Design review of the part built by this model. Coordinates are the model's own, in mm. Face numbers are marked on the shaded views. A direction names the side the tool comes from. Round coordinates to 2 decimals unless told otherwise and drop trailing zeros. Write each loop counter-clockwise with the first axis right and the second up, starting at its lowest first coordinate (ties: lowest second). Pieces come first, ordered by that corner, then holes. Notation, with made-up numbers: (-20.75, 44.5) -> (-15.75, 44.5) arc R28 ccw to (-15.75, 68.5) -> close; hole circle Ø4 at (-1, 55.25). An arc over 180 degrees is marked (long way). Write item = value, one per line. Start each with the question number.
Item 1: Add section A-A, the plane y = -7. State the section outline as (x, z) points.
Item 2: Machinability: for the marked faces 4, 5 and 6, which of the approach directions +Z, -Z, +X, -X, +Y, -Y give a long, thin tool a straight path to every point of the face, cutting with its end or side? Answer none if there is none.
Item 3: Add section C-C, the plane z = -124. State the section outline as (x, y) points, then the cut area to 3 significant figures.
Item 4: Add section B-B, the plane x = 213. State the section outline as (y, z) points.
Item 5: To check wall thickness, follow L1, parallel to Z at x = 251, y = 0; L2, parallel to Y at x = -15.5, z = -142.5; L3, parallel to Y at x = 222.5, z = -102. State the ranges of each line that lie inside material, in increasing order.
Item 6: Mouldability with a two-part tool opening along Z and no side actions: class the marked faces 1, 2 and 3 as released by +Z, released by -Z, zero draft, split by the parting line, or undercut.
Item 7: For pin 1 Ø1 at (y, z) = (-8.5, -175) entering from -X; pin 2 Ø3 at (x, y) = (177, 14.5) entering from +Z; pin 3 Ø3 at (y, z) = (3.5, -131.5) entering from -X, all flat-tipped, find the tip position at first contact; note any pin that passes through.
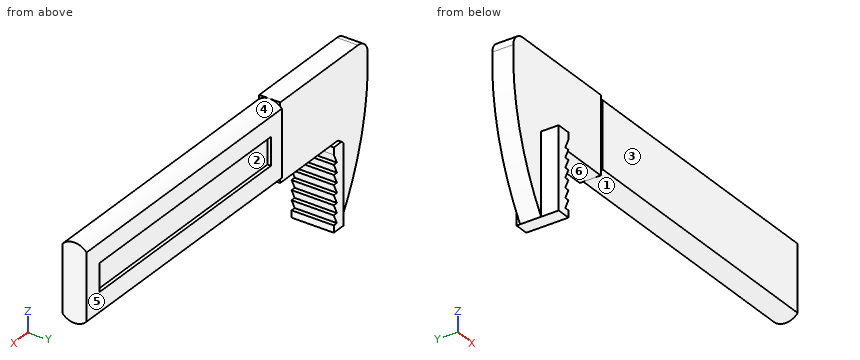
Autodesk Inventor part; units mm, degrees
ref_plane "YZ Plane" through (0, 0, 0) normal (1, 0, 0) x (0, 1, 0)
ref_plane "XZ Plane" through (0, 0, 0) normal (0, 1, 0) x (-1, 0, 0)
ref_plane "XY Plane" through (0, 0, 0) normal (0, 0, 1) x (1, 0, 0)
sketch "Sketch1" plane through (0, 0, 0) normal (0, 1, 0) x (-1, 0, 0)
  line L0 (0, -131.5012) -> (-0.0617, -190.607)
  line L1 (-41.7658, -131.5012) -> (53.7037, -131.5012) construction
  line L2 (28.2495, -75.6212) -> (-41.7658, -75.6212)
  arc A0 (-0.0617, -190.607) -> (28.2495, -75.6212) centre (-152.8189, -92.0177) ccw
  line L3 (28.2495, -75.6212) -> (-62.1692, -75.6212)
  line L4 (-62.1692, -75.6212) -> (-62.1692, -131.5012)
  line L5 (-62.1692, -131.5012) -> (0, -131.5012)
  point P0 (0, 0)
  point P1 (8.9112, -179.6369)
  point P2 (0, -75.6212)
  point P3 (-70.1734, -131.5012)
  dimension "d21" = 59.1058
  dimension "d37" = 70.0153
extrude "Extrusion1" add sketch "Sketch1" along normal blind 15.24
fillet "Fillet1" radius 10.16 1 edges at (-28.2495, 7.62, -75.6212)
sketch "Sketch4" plane through (0.0191, 12.7, -149.7788) normal (0.9999995, 0, 0.0010447) x (0.0010447, 0, -0.9999995)
  line L0 (0, -22.86) -> (0, 2.54)
  line L1 (15.9389, 2.54) -> (13.4561, 2.54) construction
  line L2 (13.4561, 2.54) -> (13.4561, 4.185) construction
  line L3 (13.6464, 2.54) -> (33.02, 2.54)
  line L4 (33.02, -22.86) -> (13.6464, -22.86)
  line L5 (-10.4713, -22.86) -> (-10.4713, 2.54) construction
  line L6 (-10.4713, -10.16) -> (33.02, -10.16) construction
  line L7 (-10.4713, -10.16) -> (11.2743, -10.16) construction
  line L8 (-18.2773, 5.1507) -> (40.826, 5.1507)
  line L9 (40.826, 5.1507) -> (40.826, -25.4707)
  line L10 (40.826, -25.4707) -> (-18.2773, -25.4707)
  line L11 (-18.2773, -25.4707) -> (-18.2773, 5.1507)
  line L12 (-18.2773, 5.1507) -> (40.826, -25.4707) construction
  line L13 (40.826, 5.1507) -> (-18.2773, -25.4707) construction
  point P0 (8.89, -10.16)
  dimension "d24" = 43.4913
  dimension "d23" = 21.7457
extrude "Extrusion4" add sketch "Sketch4" along normal blind 10.16
sketch "Sketch5" plane through (0, 17.8507, -131.5015) normal (0, 1, 0) x (0.9999995, 0, 0.0010447)
  line L0 (10.16, 0) -> (10.16, 59.1033)
  line L1 (10.16, 0) -> (10.16, 4.6168)
  line L2 (10.16, 0) -> (10.16, 6.604)
  line L3 (10.16, 59.1033) -> (10.16, 54.0318)
  line L4 (10.16, 54.0318) -> (6.8983, 54.0318)
  line L5 (6.8983, 54.0318) -> (10.16, 47.0371)
  line L6 (10.16, 3.5366) -> (10.16, 0)
  line L7 (10.16, 54.0318) -> (10.16, 59.1033)
  line L8 (10.16, 47.0371) -> (6.8983, 47.0371)
  line L9 (6.8983, 47.0371) -> (10.16, 40.0424)
  line L10 (10.16, 40.0424) -> (6.8983, 40.0424)
  line L11 (6.8983, 40.0424) -> (10.16, 33.0478)
  line L12 (10.16, 33.0478) -> (6.8983, 33.0478)
  line L13 (6.8983, 33.0478) -> (10.16, 26.0531)
  line L14 (10.16, 26.0531) -> (6.8983, 26.0531)
  line L15 (6.8983, 26.0531) -> (10.16, 19.0584)
  line L16 (10.16, 19.0584) -> (6.8983, 19.0584)
  line L17 (6.8983, 19.0584) -> (10.16, 12.0637)
  line L18 (10.16, 12.0637) -> (6.8983, 12.0637)
  line L19 (6.8983, 12.0637) -> (10.16, 5.0691)
  line L20 (10.16, 5.0691) -> (10.16, 54.0318)
  point P0 (-241.3, 27.1673)
  dimension "d30" = 5.0715
  dimension "d28" = 65
  dimension "d29" = 6.9947
extrude "Extrusion5" cut sketch "Sketch5" against normal through all
fillet "Fillet3" radius 3.175 1 edges at (0, 16.5453, -131.5015)
sketch "Sketch7" plane through (62.1692, 0, -75.6212) normal (1, 0, 0) x (0, 0, -1)
  line L0 (0, 15.24) -> (55.88, 15.24)
  line L1 (55.88, 0) -> (27.2823, 0)
  line L2 (27.94, 0) -> (41.91, 0) construction
  line L3 (55.88, 0) -> (55.88, 15.24)
  line L4 (55.88, 0) -> (27.94, 0)
  line L5 (9.7909, 0) -> (0, 0)
  line L6 (27.94, 0) -> (27.94, 15.24)
  line L7 (27.94, 15.24) -> (53.086, 15.24)
  line L8 (114.9858, 15.24) -> (9.7909, 15.24)
  arc A0 (51.9331, -1.1819) -> (51.9331, 16.4219) centre (44.0921, 7.62) ccw
  line L9 (51.9331, 16.4219) -> (51.9331, -1.1819) construction
  line L10 (51.9331, 16.4219) -> (69.5369, 16.4219) construction
  arc A1 (3.9469, 16.4219) -> (3.9469, -1.1819) centre (11.7879, 7.62) ccw
  line L11 (3.9469, 16.4219) -> (51.9331, 16.4219)
  line L12 (3.9469, -1.1819) -> (51.9331, -1.1819)
  point P0 (-75.6212, 0)
  dimension "d43" = 27.94
  dimension "d44" = 25.146
  dimension "d45" = 90
  dimension "d56" = 17.6038
extrude "Extrusion6" add sketch "Sketch7" along normal blind 203.2 contours L0 A1 L11 A0 | L0 L6 L1 A0 L12 A1 | L0 A0 L1 L6
sketch "Sketch8" plane through (62.1692, 16.4219, -79.5681) normal (0, 1, 0) x (1, 0, 0)
  line L0 (203.2, 47.9862) -> (203.2, 0) construction
  line L1 (203.2, 23.9931) -> (-91.0395, 23.9931) construction
  arc A0 (-62.1075, 111.0389) -> (-91.0395, 5.8439) centre (90.6496, 12.4496) ccw construction
  line L2 (-91.0395, 5.8439) -> (-91.0395, 27.6375) construction
  line L3 (-91.0395, 5.8439) -> (-69.2459, 5.8439) construction
  line L4 (203.2, 0) -> (56.0832, 0) construction
  line L5 (0, 0) -> (203.2, 0) construction
  line L6 (56.0832, 0) -> (56.0832, 60.6628) construction
  line L7 (-77.8013, 6.5731) -> (189.9677, 41.4131) construction
  line L8 (189.9677, 6.5731) -> (-77.8013, 41.4131) construction
  line L9 (11.3147, 13.9418) -> (189.9677, 13.9418)
  line L10 (189.9677, 13.9418) -> (189.9677, 34.0444)
  line L11 (189.9677, 34.0444) -> (11.3147, 34.0444)
  line L12 (11.3147, 34.0444) -> (11.3147, 13.9418)
  line L13 (11.3147, 13.9418) -> (189.9677, 34.0444) construction
  line L14 (189.9677, 13.9418) -> (11.3147, 34.0444) construction
  point P0 (-62.1692, -79.5681)
  point P1 (56.0832, 23.9931)
  point P2 (100.6412, 23.9931)
  dimension "d48" = 90
  dimension "d50" = 147.1168
extrude "Extrusion7" cut sketch "Sketch8" against normal blind 2.54
properties part number "Top"
Result set:
q1.outline = (0, -131.5) -> (0.06, -190.6) -> (10.22, -190.59) -> (10.22, -185.52) -> (6.95, -185.53) -> (10.21, -178.53) -> (6.95, -178.53) -> (10.2, -171.53) -> (6.94, -171.54) -> (10.19, -164.54) -> (6.93, -164.54) -> (10.19, -157.54) -> (6.93, -157.55) -> (10.18, -150.55) -> (6.92, -150.55) -> (10.17, -143.55) -> (6.91, -143.56) -> (10.17, -136.56) -> (10.16, -131.49) -> close
q2.face_4 = +Z, +X
q2.face_5 = +Z, -Z, +X, -X, +Y
q2.face_6 = -Z, +X, +Y, -Y
q3.outline = (-26.16, 0) -> (62.17, 0) -> (62.17, -1.18) -> (265.37, -1.18) -> (265.37, 16.42) -> (62.17, 16.42) -> (62.17, 15.24) -> (-26.16, 15.24) -> close
q3.area = 4,920 mm²
q4.outline = (-1.18, -127.55) arc R11.79 ccw to (16.42, -127.55) -> (16.42, -113.61) -> (13.88, -113.61) -> (13.88, -93.51) -> (16.42, -93.51) -> (16.42, -79.57) arc R11.79 ccw to (-1.18, -79.57) -> close
q5.L1 = -128.71 to -78.42
q5.L2 = 0 to 15.24
q5.L3 = -1.18 to 13.88
q6.face_1 = released by -Z
q6.face_2 = undercut
q6.face_3 = zero draft
q7.pin_1 = 0.04
q7.pin_2 = -76.92
q7.pin_3 = -24.98
